The listing builds one solid part. Answer for the finished solid, in the listing's coordinates (mm). Face numbers are marked on the shaded views. A direction names the side the tool comes from. Give positions to 0.01 mm unless a question says otherwise; leave off trailing zeros. Write each loop counter-clockwise with the first axis right and the second up, starting at its lowest first coordinate (ties: lowest second). Pieces come first, ordered by that corner, then holes. Notation, with made-up numbers: M 13.25,52 L 69.25,52 A15 cw 69.25,81 Z; hole C 77,61.25 d9. An arc over 180 degrees is marked long. Return JSON: item names as keys, results as strings.
from build123d import *

# Parameters (mm, degrees)
BOX003_W      = 70
BOX003_H      = 70
BOX003_DEPTH  = 150
BOX001_W      = 10
BOX001_H      = 10
BOX001_DEPTH  = 14
ARRAY_X_COUNT = 5
ARRAY_X_PITCH = 20
ARRAY_Y_COUNT = 5
ARRAY_Y_PITCH = 20
BOX002_W      = 110
BOX002_H      = 110
BOX002_DEPTH  = 10
BOX_W         = 90
BOX_H         = 90
BOX_DEPTH     = 150


with BuildPart() as cube003:
    # Box003 → Box003 (new body)
    with BuildSketch(Plane(origin=(10, 10, 3), x_dir=(1, 0, 0), z_dir=(0, 0, 1))):
        with Locations((35, 35)):
            Rectangle(BOX003_W, BOX003_H)
    extrude(amount=BOX003_DEPTH)


with BuildPart() as array:
    # Box001 → Box001 (new body)
    with BuildSketch(Plane.XY):
        with Locations((5, 5)):
            Rectangle(BOX001_W, BOX001_H)
    extrude(amount=BOX001_DEPTH)

    # Array X: Array ×5


with BuildPart() as array_1:
    add(array.part)
    with Locations(*[(i * ARRAY_X_PITCH, 0, 0) for i in range(1, ARRAY_X_COUNT)]):
        add(array.part)

    # Array Y: Array ×5


with BuildPart() as array_2:
    add(array_1.part)
    with Locations(*[(0, i * ARRAY_Y_PITCH, 0) for i in range(1, ARRAY_Y_COUNT)]):
        add(array_1.part)


with BuildPart() as cut:
    # Box002 → Box002 (new body)
    with BuildSketch(Plane(origin=(-10, -9, 0), x_dir=(1, 0, 0), z_dir=(0, 0, 1))):
        with Locations((55, 55)):
            Rectangle(BOX002_W, BOX002_H)
    extrude(amount=BOX002_DEPTH)

    # Cut: cut Array
    add(array_2.part, mode=Mode.SUBTRACT)


with BuildPart() as cut_1:
    # Cut placement: moved
    add(cut.part.moved(Location((0, 0, 140))))


with BuildPart() as cut002:
    # Box → Box (new body)
    with BuildSketch(Plane.XY):
        with Locations((45, 45)):
            Rectangle(BOX_W, BOX_H)
    extrude(amount=BOX_DEPTH)

    # Cut001: cut Cut
    add(cut_1.part, mode=Mode.SUBTRACT)

    # Cut002: cut Cube003
    add(cube003.part, mode=Mode.SUBTRACT)


solid = cut002.part
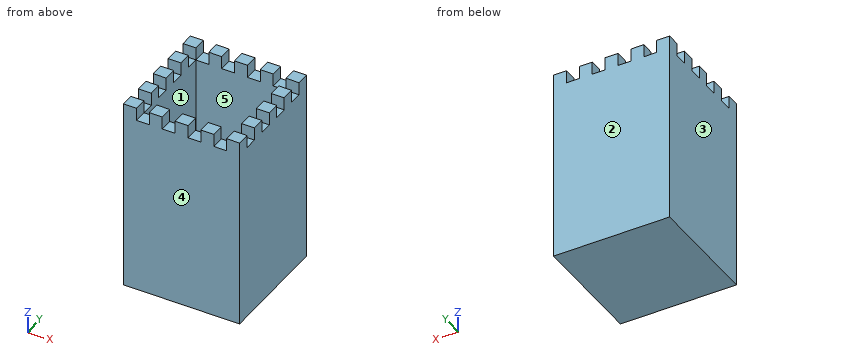
Item 1: A cutting plane is placed at D-D, the plane x = 8. Write down the section's boundary in (y, z).
Geometry results:
{"outline": "M 0,0 L 90,0 L 90,150 L 80,150 L 80,140 L 70,140 L 70,150 L 60,150 L 60,140 L 50,140 L 50,150 L 40,150 L 40,140 L 30,140 L 30,150 L 20,150 L 20,140 L 10,140 L 10,150 L 0,150 Z"}
Item 2: A cutting plane is placed at B-B, the plane x = 35.5. Write down the section's boundary in (y, z), plus the area to 3 significant figures.
Geometry results:
{"outline": "M 0,0 L 90,0 L 90,140 L 80,140 L 80,3 L 10,3 L 10,140 L 0,140 Z", "area": "3,010 mm2"}
Item 3: Determine the mould class of the marked faces 1, 2 and 3 for opening direction Y: +Y half, -Y half, draft (parallel to the pull), parting line (faces both ways), or undercut.
Geometry results:
{"face 1": "undercut", "face 2": "+Y half", "face 3": "draft"}
Item 4: A cutting plane is placed at A-A, the plane z = 46.5. Write down the section's boundary in (x, y).
Geometry results:
{"outline": "M 0,0 L 90,0 L 90,90 L 0,90 Z; hole M 10,10 L 80,10 L 80,80 L 10,80 Z"}
Item 5: Find the intervals of material crossed by line 1 (X direction, y = 30.5, z = 25.5); line 2 (Z direction, x = 59, y = 61), in increasing order.
Geometry results:
{"line 1": "x = 0 to 10, 80 to 90", "line 2": "z = 0 to 3"}
Item 6: Given pin 1 Ø3 at (x, y) = (4, 72.5) entering from +Z, flat-ended and moving along its own axis, determine where the tip first touches the part or whether it passes through.
Geometry results:
{"pin 1": "stops at z = 140"}
Item 7: Which of the six approach directions +Z, -Z, +X, -X, +Y, -Y give full straight-line access (tool end or side, diameter ignored) to the marked faces 4 and 5?
Geometry results:
{"face 4": "+Z, -Z, +X, -X, -Y", "face 5": "+Z"}
